Could you check a few things on this model? Use its own coordinates, in mm. A direction names the side the tool comes from. Coordinates: 2 decimals unless noted, no trailing zeros. Write each loop counter-clockwise with the first axis right and the second up, starting at its lowest first coordinate (ties: lowest second). Pieces come first, ordered by that corner, then holes. Notation, with made-up numbers: M 5.5,-16.75 L 45.5,-16.75 A17 cw 45.5,-4.75 Z; hole C 46.5,-4.5 d7. An arc over 180 degrees is marked long. Write item = value, one per line.
```python
from build123d import *

# Parameters (mm, degrees)
SKETCH1_W           = 4
SKETCH1_H           = 5
BOSS_EXTRUDE1_DEPTH = 30
SKETCH2_W           = 5
SKETCH2_H           = 5
BOSS_EXTRUDE2_DEPTH = 10
SKETCH3_R           = 1.25
CUT_EXTRUDE1_DEPTH  = 33.015621187
CUT_EXTRUDE2_DEPTH  = 34.481338086


with BuildPart() as part:
    # Sketch1 → Boss-Extrude1 (new body)
    with BuildSketch(Plane(origin=(0, 0, 0), x_dir=(1, 0, 0), z_dir=(0, 1, 0))):
        with Locations((2, -2.5)):
            Rectangle(SKETCH1_W, SKETCH1_H)
    extrude(amount=BOSS_EXTRUDE1_DEPTH)

    # Sketch2 → Boss-Extrude2 (add)
    with BuildSketch(Plane(origin=(4, 0, 0), x_dir=(0, 0, -1), z_dir=(1, 0, 0))):
        with Locations((-2.5, 15)):
            Rectangle(SKETCH2_W, SKETCH2_H)
    extrude(amount=BOSS_EXTRUDE2_DEPTH)

    # Sketch3 → Cut-Extrude1 (cut, through all)
    with BuildSketch(Plane(origin=(4, 0, 0), x_dir=(0, 0, -1), z_dir=(1, 0, 0))):
        with Locations((-2.5, 25)):
            Circle(SKETCH3_R)
        with Locations(Location((-2.5, 5, 0), (0, 0, 180))):
            Circle(SKETCH3_R)
    extrude(amount=-CUT_EXTRUDE1_DEPTH, mode=Mode.SUBTRACT)

    # Sketch4 → Cut-Extrude2 (cut, through all)
    with BuildSketch(Plane(origin=(0, 0, 0), x_dir=(1, 0, 0), z_dir=(0, 1, 0))):
        with BuildLine():
            Line((8, 0), (10, 0))
            ThreePointArc((10, 0), (9, -1), (8, 0))
        make_face()
    extrude(amount=CUT_EXTRUDE2_DEPTH, mode=Mode.SUBTRACT)


solid = part.part
```
Item 1: If I drill on line 1 along Y through (x, z) = (2.35, 2.5); line 2 along Y through (x, z) = (5, 3); line 3 along X through (y, z) = (7.5, 3.8), over which ranges is the centre line in solid material (lowest first)?
Numbers:
line_1 = 0 to 3.75, 6.25 to 23.75, 26.25 to 30
line_2 = 12.5 to 17.5
line_3 = 0 to 4
Item 2: Imagine slicing it at A-A (z = 2.5). Write out the boundary of the cut face in (x, y).
Numbers:
outline = M 0,0 L 4,0 L 4,3.75 L 0,3.75 Z; M 0,6.25 L 4,6.25 L 4,12.5 L 14,12.5 L 14,17.5 L 4,17.5 L 4,23.75 L 0,23.75 Z; M 0,26.25 L 4,26.25 L 4,30 L 0,30 Z
Item 3: Imagine slicing it at D-D (y = 20.5). Write out the boundary of the cut face in (x, z).
Numbers:
outline = M 0,0 L 4,0 L 4,5 L 0,5 Z
Item 4: I'm going to push flat-ended pins straight in: P1, Ø1.5, axis at x = 2, y = 13.5, coming from the -Z side; P2, Ø2, axis at y = 6, z = 1, coming from the +X side; P3, Ø1.5, axis at x = 8.5, z = 2.5, coming from the +Y side; P4, Ø1.5, axis at x = 10.5, z = 2.5, coming from the -Y side. Where does each tip first touch, or does it pass through?
Numbers:
P1 = 0
P2 = 4
P3 = 17.5
P4 = 12.5
Item 5: Imagine slicing it at B-B (x = 3.5). Write out the boundary of the cut face in (y, z), and give its area (3 significant figures).
Numbers:
outline = M 0,0 L 30,0 L 30,5 L 0,5 Z; hole C 5,2.5 d2.5; hole C 25,2.5 d2.5
area = 140 mm²
Item 6: If we mould it in two halves opening along X, with no side actions, what happens to faces 1 (the face through (9, 15, 1)), 2 (the face through (14, 15, 3)), 3 (the face through (0, 15, 3)), 4 (the face through (2.028, 6.109, 3.077))? For each: pulls with the +X half, pulls with the -X half, needs draft (parallel to the pull), parting line crosses it, or undercut.
Numbers:
face_1 = undercut
face_2 = pulls with the +X half
face_3 = pulls with the -X half
face_4 = needs draft
Item 7: Imagine slicing it at C-C (y = 25). Write out the boundary of the cut face in (x, z), and give its area (3 significant figures).
Numbers:
outline = M 0,0 L 4,0 L 4,1.25 L 0,1.25 Z; M 0,3.75 L 4,3.75 L 4,5 L 0,5 Z
area = 10.0 mm²
Item 8: For faces 5 (the face through (4, 6, 4)), 6 (the face through (4, 23.7, 3.1)), 7 (the face through (2, 30, 2)), which set-ups out of +Z, -Z, +X, -X, +Y, -Y let a thin tool reach every point of the face, with its end or its side?
Numbers:
face_5 = +Z, -Z, +X, -Y
face_6 = +Z, -Z, +X, +Y
face_7 = +Z, -Z, +X, -X, +Y
